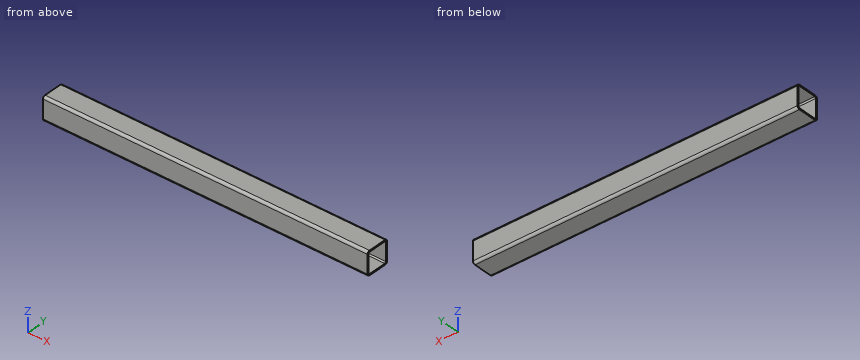
from build123d import *

# Parameters (mm, degrees)
F2_DEPTH = 444.5
F3_ANGLE = 90


# Not quite as in the source:
# - a variable given as a bare number and used for a length is read in inches; the dataset says mm whatever the document's units were


with BuildPart() as f2:
    # F0 (on Top) → F2 (new body)
    with BuildSketch(Plane.XY):
        with BuildLine():
            Line((-12.573, -15.875), (12.573, -15.875))
            ThreePointArc((12.573, -15.875), (14.9078665915, -14.9078665915), (15.875, -12.573))
            Line((15.875, -12.573), (15.875, 12.573))
            ThreePointArc((15.875, 12.573), (14.9078665915, 14.9078665915), (12.573, 15.875))
            Line((12.573, 15.875), (-12.573, 15.875))
            ThreePointArc((-12.573, 15.875), (-14.9078665915, 14.9078665915), (-15.875, 12.573))
            Line((-15.875, 12.573), (-15.875, -12.573))
            ThreePointArc((-15.875, -12.573), (-14.9078665915, -14.9078665915), (-12.573, -15.875))
        make_face()
        with BuildLine():
            Line((-12.573, 14.224), (12.573, 14.224))
            ThreePointArc((12.573, 14.224), (13.7404332957, 13.7404332957), (14.224, 12.573))
            Line((14.224, 12.573), (14.224, -12.573))
            ThreePointArc((14.224, -12.573), (13.7404332957, -13.7404332957), (12.573, -14.224))
            Line((12.573, -14.224), (-12.573, -14.224))
            ThreePointArc((-12.573, -14.224), (-13.7404332957, -13.7404332957), (-14.224, -12.573))
            Line((-14.224, -12.573), (-14.224, 12.573))
            ThreePointArc((-14.224, 12.573), (-13.7404332957, 13.7404332957), (-12.573, 14.224))
        make_face(mode=Mode.SUBTRACT)
    extrude(amount=F2_DEPTH)


with BuildPart() as f2_1:
    # F3: moved
    add(f2.part.rotate(Axis((-15.875, 0, 444.5), (0, 1, 0)), F3_ANGLE))


solid = f2_1.part
Check sheet for the modelled part. Datum: model origin and axes. Units: mm. Round coordinates to 2 decimals unless told otherwise and drop trailing zeros. Loops run counter-clockwise (first coordinate to the right, second up) from the corner with the lowest first, then second, coordinate; pieces in that order, holes last. Notation, with made-up numbers: M -28,29 L -4,29 A11 ccw -4,36 Z; hole C 81.5,49 d7. An arc over 180 degrees is marked long. One line per question, with ' | ' between items. Start each with the question number.
Item 1: Section check A-A (y = -5.5). Record the boundary of the cut face in (x, z) (3 decimals), and give its area (3 significant figures).
Item 2: Section check B-B (x = -175). Record the boundary of the cut face in (y, z) (3 decimals).
Item 3: Scan lines: probe 1 along Z at (x, y) = (-255, -12); probe 2 along Y at (x, z) = (-287.5, 438.5) (3 decimals). Record each from-to range of solid material in increasing order.
Item 4: Section check C-C (z = 422.5). Record the boundary of the cut face in (x, y) (3 decimals).
Worked out:
1) outline: M -460.375,412.75 L -15.875,412.75 L -15.875,414.401 L -460.375,414.401 Z; M -460.375,442.849 L -15.875,442.849 L -15.875,444.5 L -460.375,444.5 Z | area: 1,470 mm^2
2) outline: M -15.875,416.052 A3.302 ccw -12.573,412.75 L 12.573,412.75 A3.302 ccw 15.875,416.052 L 15.875,441.198 A3.302 ccw 12.573,444.5 L -12.573,444.5 A3.302 ccw -15.875,441.198 Z; hole M -14.224,416.052 A1.651 ccw -12.573,414.401 L 12.573,414.401 A1.651 ccw 14.224,416.052 L 14.224,441.198 A1.651 ccw 12.573,442.849 L -12.573,442.849 A1.651 ccw -14.224,441.198 Z
3) probe 1: 412.75 to 414.4, 442.85 to 444.5 | probe 2: -15.875 to -14.224, 14.224 to 15.875
4) outline: M -460.375,-15.875 L -15.875,-15.875 L -15.875,-14.224 L -460.375,-14.224 Z; M -460.375,14.224 L -15.875,14.224 L -15.875,15.875 L -460.375,15.875 Z
